```python
from build123d import *

# Parameters (mm, degrees)
F2_T     = -1.3462
F0_W     = 21.1836
F0_H     = 7.239
F4_R     = 2.4003
F5_DEPTH = 4.4958
F7_DEPTH = 2.794
F8_W     = 2.2705799568
F8_H     = 2.54
F8_W_2   = 2.7586200432
F9_DEPTH = 10.16


with BuildPart() as f1:
    # F0 (on Front) → F1 (revolve)
    with BuildSketch(Plane.XZ):
        Polygon((0, 7.239), (0, 0), (16.5415440198, 0), (16.5415440198, 13.0302), align=None)
    revolve(axis=Axis((-10.5918, 0, 0), (-1, 0, 0)))

    # F2
    f2_openings = [f1.faces().sort_by_distance(p)[0] for p in [
        (16.541544, 0, 0),
    ]]
    offset(amount=F2_T, openings=f2_openings)

    # F0 (on Front) → F3 (revolve)
    with BuildSketch(Plane.XZ):
        with Locations((-10.5918, 3.6195)):
            Rectangle(F0_W, F0_H)
    revolve(axis=Axis((-10.5918, 0, 0), (-1, 0, 0)))

    # F4 (on face) → F5 (join)
    with BuildSketch(Plane(origin=(-21.1836, 0, 0), x_dir=(0, -1, 0), z_dir=(-1, 0, 0))):
        Circle(F4_R)
    extrude(amount=F5_DEPTH)

    # F6 (on Top) → F7 (join, symmetric)
    with BuildSketch(Plane.XY):
        with BuildLine():
            Line((-8.1743659384, 13.9954), (-8.1743659384, 4.5510675645))
            Line((-8.1743659384, 4.5510675645), (-2.6625659384, 4.5510675645))
            Line((-2.6625659384, 4.5510675645), (-2.6625659384, 13.9954))
            ThreePointArc((-2.6625659384, 13.9954), (-5.4184659384, 11.2395), (-8.1743659384, 13.9954))
        make_face()
        with BuildLine():
            ThreePointArc((-2.6625659384, 13.9954), (-5.4184659384, 16.7513), (-8.1743659384, 13.9954))
            Line((-8.1743659384, 13.9954), (-6.5106659384, 13.9954))
            ThreePointArc((-6.5106659384, 13.9954), (-5.4184659384, 15.0876), (-4.3262659384, 13.9954))
            Line((-4.3262659384, 13.9954), (-2.6625659384, 13.9954))
        make_face()
        with BuildLine():
            Line((-6.5106659384, 13.9954), (-8.1743659384, 13.9954))
            ThreePointArc((-8.1743659384, 13.9954), (-5.4184659384, 11.2395), (-2.6625659384, 13.9954))
            Line((-2.6625659384, 13.9954), (-4.3262659384, 13.9954))
            ThreePointArc((-4.3262659384, 13.9954), (-5.4184659384, 12.9032), (-6.5106659384, 13.9954))
        make_face()
    extrude(amount=F7_DEPTH, both=True)

    # F8 (on face) → F9 (cut)
    with BuildSketch(Plane(origin=(-8.1743659384, 0, 0), x_dir=(0, -1, 0), z_dir=(-1, 0, 0))):
        with Locations((-12.8601100216, 0)):
            Rectangle(F8_W, F8_H)
        with Locations((-15.3747100216, 0)):
            Rectangle(F8_W_2, F8_H)
    extrude(amount=-F9_DEPTH, mode=Mode.SUBTRACT)

    # F10 (on Front) → F11 (revolve)
    with BuildSketch(Plane.XZ):
        with BuildLine():
            Line((7.4050883165, 4.5414811682), (0, 2.8554751822))
            Line((0, 2.8554751822), (0, 0))
            Line((0, 0), (8.9534996077, 0))
            ThreePointArc((8.9534996077, 0), (8.4175012065, 1.2725301509), (7.0793638567, 1.6131409325))
            Line((7.0793638567, 1.6131409325), (7.4050883165, 4.5414811682))
        make_face()
    revolve(axis=Axis((8.2707720099, 0, 0), (-1, 0, 0)))


solid = f1.part
```
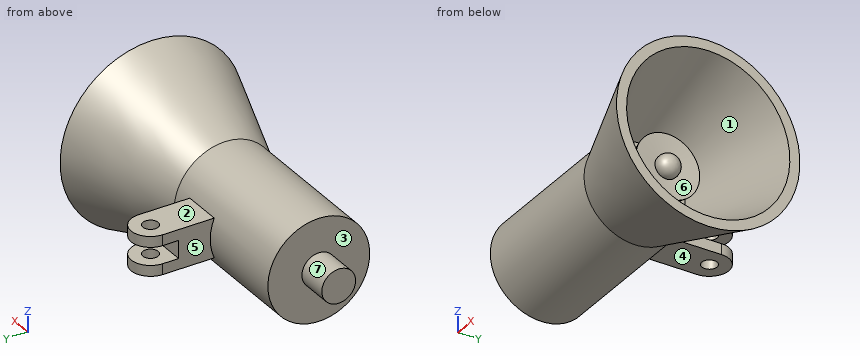
Build history of the part. All positions in model axes, mm. Face numbers are marked on the shaded views. A direction names the side the tool comes from. Give positions to 0.01 mm unless a question says otherwise; leave off trailing zeros.
1) Band-saw the part on A-A on y = 12.25. State how many separate pieces and enclosed holes the cut face has, then the cut area to 3 significant figures.
Values follow:
separate pieces: 3
enclosed holes: 0
area: 29.9 mm2
2) Drop flat-ended pins along their axis: P1, Ø10, axis at x = -15, y = 5, coming from the +Z side; P2, Ø1.7, axis at x = -5.5, y = 10.5, coming from the +Z side; P3, Ø2, axis at x = -9, y = 6, coming from the +Z side; P4, Ø6, axis at y = 11.5, z = 0, coming from the +X side. Give the stop position or say it passes through.
Values follow:
P1: stops at z = 7.24
P2: stops at z = 2.79
P3: stops at z = 5.23
P4: stops at x = 16.54
3) Probe line 1 along Y through (x, z) = (7.5, 0.75); line 2 along Z through (x, y) = (3, -2.25); line 3 along Z through (x, y) = (6.5, -5). List the from-to ranges inside material, lowest first.
Values follow:
line 1: y = -9.84 to -8.41, -1.46 to 1.46, 8.41 to 9.84
line 2: z = -7.98 to -6.48, -2.73 to 2.73, 6.48 to 7.98
line 3: z = -8.09 to -6.36, 6.36 to 8.09
4) 3-axis set-ups, long thin cutter, end or side, ignore diameter. For the marked faces 1, 2, 3 and 4: which of +Z, -Z, +X, -X, +Y, -Y reach the whole face in a straight line?
Values follow:
face 1: +X
face 2: +Z, -X, +Y
face 3: -X
face 4: -Z, -X, +Y
5) Two-plate mould, pull along Z, no slides. Class the marked faces 5, 6 and 7: released by +Z, released by -Z, zero draft, split by the parting line, or undercut.
Values follow:
face 5: zero draft
face 6: undercut
face 7: split by the parting line
